Here's how the part is built. I have some questions about the finished solid (model axes, mm). Face numbers are marked on the shaded views. A direction names the side the tool comes from. Coordinates: 2 decimals unless noted, no trailing zeros. Order: outer loops, then holes, each group sorted by start corner. A loop starts at its lowest first (then second) coordinate and runs counter-clockwise, first axis right, second up. Notation, with made-up numbers: (6, 29.25) - (63, 29.25) arc R33 cw to (63, 64.25) - close; hole circle Ø3 at (-20, 34). An arc over 180 degrees is marked (long way). Answer as CSV lines item,"result". Start each with the question number.
Q1. For the marked faces 3 and 4, which set-ups out of +Z, -Z, +X, -X, +Y, -Y let a thin tool reach every point of the face, with its end or its side?
Q2. Suppose I cut it at B-B (z = -20). Please give me the cut outline in (x, y).
Q3. Thinking about a two-plate mould opening in Z: for the marked faces 1 and 2, which applies, released by +Z, released by -Z, zero draft, split by the parting line, or undercut?
Q4. Suppose I cut it at C-C (x = -1.5). Please give me the cut outline in (y, z).
Q5. I need wall thicknesses on line 1 (Z direction, x = 54, y = 0.75); line 2 (Z direction, x = 26, y = 3.75); line 3 (Z direction, x = -33, y = 3.5). Which ranges of each line are inside material? Lowest first, please.
Q6. Suppose I cut it at A-A (x = -64.5). Please give me the cut outline in (y, z), then the cut area to 3 significant figures.
Q7. Suppose I cut it at D-D (x = 125). Please give me the cut outline in (y, z) (3 decimals).
Q8. For pin 1 Ø6 at (x, z) = (143.5, -4.5) entering from -Y; pin 2 Ø1.9 at (y, z) = (3.5, 83.5) entering from +X; pin 3 Ø5 at (x, z) = (125.5, -4) entering from +Y, each with a flat end and sliding along its axis, tell me the tip position at first contact or that it passes through.
from build123d import *

# Parameters (mm, degrees)
SALIENTE_EXTRUIR1_DEPTH = 6.35
CROQUIS2_R              = 1.825
CROQUIS2_W              = 63.849825594
CROQUIS2_H              = 10
CROQUIS2_W_2            = 24.299825594
CORTAR_EXTRUIR1_DEPTH   = 220.409920137
CROQUIS4_W              = 45
CROQUIS4_H              = 84.1
CORTAR_EXTRUIR3_DEPTH   = 1.5
CROQUIS5_R              = 1.75
CORTAR_EXTRUIR4_DEPTH   = 220.371632292
CROQUIS7_W              = 45
CROQUIS7_H              = 2.275
CORTAR_EXTRUIR5_DEPTH   = 1.5
CROQUIS9_W              = 125
CROQUIS9_H              = 146
CORTAR_EXTRUIR7_DEPTH   = 4.3
CROQUIS10_R             = 2.8
CORTAR_EXTRUIR8_DEPTH   = 4.35
CORTAR_EXTRUIR12_DEPTH  = 220.409920137
CORTAR_EXTRUIR15_DEPTH  = 1.5
CROQUIS19_W             = 7.395174406
CROQUIS19_H             = 10
CORTAR_EXTRUIR16_DEPTH  = 220.409920137
CROQUIS20_W             = 60.600000004
CROQUIS20_H             = 97.5
CORTAR_EXTRUIR17_DEPTH  = 4
CROQUIS21_R             = 1.825
CORTAR_EXTRUIR18_DEPTH  = 220.354486059
CROQUIS25_W             = 35.4
CROQUIS25_H             = 12
CORTAR_EXTRUIR21_DEPTH  = 220.409920137
CORTAR_EXTRUIR22_DEPTH  = 220.36016173
CROQUIS28_R             = 1.825
CORTAR_EXTRUIR24_DEPTH  = 220.409920137


with BuildPart() as part:
    # Croquis1 → Saliente-Extruir1 (new body)
    with BuildSketch(Plane(origin=(0, 0, 0), x_dir=(1, 0, 0), z_dir=(0, 1, 0))):
        with BuildLine():
            Line((0, 0), (200, 0))
            Line((200, 0), (200, 15.2))
            ThreePointArc((200, 15.2), (197.701163079, 20.938172036), (191.9990235, 23.3249845))
            ThreePointArc((191.9990235, 23.3249845), (148.666739026, 44.032184001), (120.7781513, 83.1307986))
            ThreePointArc((120.7781513, 83.1307986), (113.982057966, 88.196272982), (105.7, 90))
            Line((105.7, 90), (0, 90))
            Line((0, 90), (-79, 90))
            ThreePointArc((-79, 90), (-84.638146896, 87.675499941), (-86.999825594, 82.052824894))
            Line((-86.999825594, 82.052824894), (-86.999825594, 41.494023494))
            ThreePointArc((-86.999825594, 41.494023494), (-92.052704294, 29.329564667), (-102.353503833, 21.119864881))
            ThreePointArc((-102.353503833, 21.119864881), (-108.040391417, 18.79326931), (-110.4, 13.12))
            Line((-110.4, 13.12), (-110.4, 0))
            Line((-110.4, 0), (0, 0))
        make_face()
    extrude(amount=SALIENTE_EXTRUIR1_DEPTH)

    # Simetría2: part across plane


with BuildPart() as part_1:
    add(part.part)
    add(part.part.mirror(Plane(origin=(0, 6.35, 0), x_dir=(1, 0, 0), z_dir=(0, 0, -1))))

    # Croquis2 → Cortar-Extruir1 (cut, through all)
    with BuildSketch(Plane(origin=(0, 6.35, 0), x_dir=(1, 0, 0), z_dir=(0, 1, 0))):
        with Locations(Location((68.5, 81.35, 0), (0, 0, 270))):
            Circle(CROQUIS2_R)
        with Locations(Location((-16.05, 81.35, 0), (0, 0, 270))):
            Circle(CROQUIS2_R)
        with Locations(Location((68.5, -81.35, 0), (0, 0, 90))):
            Circle(CROQUIS2_R)
        with Locations(Location((-16.05, -81.35, 0), (0, 0, 90))):
            Circle(CROQUIS2_R)
        with Locations((29.925087203, -81.35)):
            Rectangle(CROQUIS2_W, CROQUIS2_H)
        with Locations((-34.849912797, -81.35)):
            Rectangle(CROQUIS2_W_2, CROQUIS2_H)
        with Locations((87.299912797, -81.35)):
            Rectangle(CROQUIS2_W_2, CROQUIS2_H)
        with Locations((-34.849912797, 81.35)):
            Rectangle(CROQUIS2_W_2, CROQUIS2_H)
        with Locations((29.925087203, 81.35)):
            Rectangle(CROQUIS2_W, CROQUIS2_H)
        with Locations((87.299912797, 81.35)):
            Rectangle(CROQUIS2_W_2, CROQUIS2_H)
    extrude(amount=-CORTAR_EXTRUIR1_DEPTH, mode=Mode.SUBTRACT)

    # Croquis4 → Cortar-Extruir3 (cut)
    with BuildSketch(Plane(origin=(0, 6.35, 0), x_dir=(1, 0, 0), z_dir=(0, 1, 0))):
        with Locations((127.5, 0)):
            Rectangle(CROQUIS4_W, CROQUIS4_H)
    extrude(amount=-CORTAR_EXTRUIR3_DEPTH, mode=Mode.SUBTRACT)

    # Croquis5 → Cortar-Extruir4 (cut, through all)
    with BuildSketch(Plane(origin=(0, 4.85, 0), x_dir=(1, 0, 0), z_dir=(0, 1, 0))):
        with Locations(Location((147.25, 35.6, 0), (0, 0, 270))):
            Circle(CROQUIS5_R)
        with Locations(Location((107.75, 35.6, 0), (0, 0, 90))):
            Circle(CROQUIS5_R)
        with Locations(Location((147.25, -35.6, 0), (0, 0, 90))):
            Circle(CROQUIS5_R)
        with Locations(Location((107.75, -35.6, 0), (0, 0, 270))):
            Circle(CROQUIS5_R)
    extrude(amount=-CORTAR_EXTRUIR4_DEPTH, mode=Mode.SUBTRACT)

    # Croquis7 → Cortar-Extruir5 (cut)
    with BuildSketch(Plane(origin=(0, 6.35, 0), x_dir=(1, 0, 0), z_dir=(0, 1, 0))):
        with Locations((127.5, 43.1875)):
            Rectangle(CROQUIS7_W, CROQUIS7_H)
    extrude(amount=-CORTAR_EXTRUIR5_DEPTH, mode=Mode.SUBTRACT)

    # Croquis9 → Cortar-Extruir7 (cut)
    with BuildSketch(Plane(origin=(0, 6.35, 0), x_dir=(1, 0, 0), z_dir=(0, 1, 0))):
        with Locations((36.10017441, 0)):
            Rectangle(CROQUIS9_W, CROQUIS9_H)
    extrude(amount=-CORTAR_EXTRUIR7_DEPTH, mode=Mode.SUBTRACT)

    # Croquis10 → Cortar-Extruir8 (cut)
    with BuildSketch(Plane.XZ):
        with Locations(Location((-16.05, 81.35, 0), (0, 0, 270))):
            Circle(CROQUIS10_R)
        with Locations(Location((-16.05, -81.35, 0), (0, 0, 90))):
            Circle(CROQUIS10_R)
        with Locations(Location((68.5, -81.35, 0), (0, 0, 270))):
            Circle(CROQUIS10_R)
        with Locations(Location((68.5, 81.35, 0), (0, 0, 90))):
            Circle(CROQUIS10_R)
    extrude(amount=-CORTAR_EXTRUIR8_DEPTH, mode=Mode.SUBTRACT)

    # Croquis16 → Cortar-Extruir12 (cut, through all)
    with BuildSketch(Plane(origin=(0, 6.35, 0), x_dir=(1, 0, 0), z_dir=(0, 1, 0))):
        Polygon((-86.999825594, 41.494023494), (-110.4, 41.494023494), (-110.4, 13.12), (-110.4, -13.12), (-110.4, -41.494023494), (-86.999825594, -41.494023494), align=None)
    extrude(amount=-CORTAR_EXTRUIR12_DEPTH, mode=Mode.SUBTRACT)

    # Croquis18 → Cortar-Extruir15 (cut)
    with BuildSketch(Plane(origin=(0, 6.35, 0), x_dir=(1, 0, 0), z_dir=(0, 1, 0))):
        Polygon((105, 44.325), (103, 44.325), (103, -44.05), (150, -44.05), (150, -42.05), (105, -42.05), align=None)
    extrude(amount=-CORTAR_EXTRUIR15_DEPTH, mode=Mode.SUBTRACT)

    # Croquis19 → Cortar-Extruir16 (cut, through all)
    with BuildSketch(Plane(origin=(0, 6.35, 0), x_dir=(1, 0, 0), z_dir=(0, 1, 0))):
        with Locations((-5.697412797, 81.35)):
            Rectangle(CROQUIS19_W, CROQUIS19_H)
        with Locations((-5.697412797, -81.35)):
            Rectangle(CROQUIS19_W, CROQUIS19_H)
    extrude(amount=-CORTAR_EXTRUIR16_DEPTH, mode=Mode.SUBTRACT)

    # Croquis20 → Cortar-Extruir17 (cut)
    with BuildSketch(Plane(origin=(0, 6.35, 0), x_dir=(1, 0, 0), z_dir=(0, 1, 0))):
        with Locations((-56.699825592, 0)):
            Rectangle(CROQUIS20_W, CROQUIS20_H)
    extrude(amount=-CORTAR_EXTRUIR17_DEPTH, mode=Mode.SUBTRACT)

    # Croquis21 → Cortar-Extruir18 (cut, through all)
    with BuildSketch(Plane(origin=(0, 2.35, 0), x_dir=(1, 0, 0), z_dir=(0, 1, 0))):
        with Locations(Location((-77.999825594, 41.75, 0), (0, 0, 270))):
            Circle(CROQUIS21_R)
        with Locations(Location((-35.999825594, 41.75, 0), (0, 0, 270))):
            Circle(CROQUIS21_R)
        with Locations(Location((-35.999825594, -41.75, 0), (0, 0, 270))):
            Circle(CROQUIS21_R)
        with Locations(Location((-77.999825594, -41.75, 0), (0, 0, 270))):
            Circle(CROQUIS21_R)
    extrude(amount=-CORTAR_EXTRUIR18_DEPTH, mode=Mode.SUBTRACT)

    # Croquis25 → Cortar-Extruir21 (cut, through all)
    with BuildSketch(Plane.XZ):
        with Locations((-49.699825594, 58.76)):
            Rectangle(CROQUIS25_W, CROQUIS25_H)
        with Locations((-49.699825594, -58.76)):
            Rectangle(CROQUIS25_W, CROQUIS25_H)
    extrude(amount=-CORTAR_EXTRUIR21_DEPTH, mode=Mode.SUBTRACT)

    # Croquis26 → Cortar-Extruir22 (cut, through all)
    with BuildSketch(Plane(origin=(0, 2.05, 0), x_dir=(1, 0, 0), z_dir=(0, 1, 0))):
        Polygon((-11.39982559, 71.5), (-11.39982559, 58), (-24.89982559, 58), (-24.89982559, -58), (-11.39982559, -58), (-11.39982559, -71.5), (83.60017441, -71.5), (83.60017441, -58), (97.10017441, -58), (97.10017441, 58), (83.60017441, 58), (83.60017441, 71.5), align=None)
    extrude(amount=-CORTAR_EXTRUIR22_DEPTH, mode=Mode.SUBTRACT)

    # Croquis28 → Cortar-Extruir24 (cut, through all)
    with BuildSketch(Plane(origin=(0, 6.35, 0), x_dir=(1, 0, 0), z_dir=(0, 1, 0))):
        with Locations(Location((-75.199825594, -62.81, 0), (0, 0, 270))):
            Circle(CROQUIS28_R)
        with Locations(Location((-58.699825594, -86, 0), (0, 0, 270))):
            Circle(CROQUIS28_R)
        with Locations(Location((-75.199825594, 62.81, 0), (0, 0, 90))):
            Circle(CROQUIS28_R)
        with Locations(Location((-58.699825594, 86, 0), (0, 0, 90))):
            Circle(CROQUIS28_R)
    extrude(amount=-CORTAR_EXTRUIR24_DEPTH, mode=Mode.SUBTRACT)


solid = part_1.part
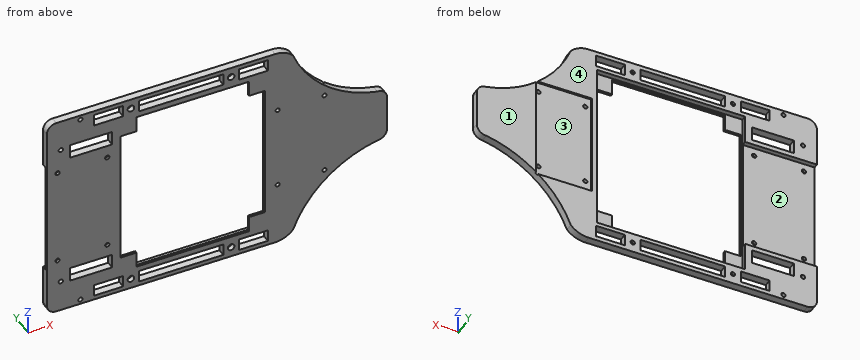
Here are the results:
1,face 3,"+Y"
1,face 4,"+Z, -Z, +X, -X, +Y"
2,outline,"(-87, 0) - (-24.9, 0) - (-24.9, 2.05) - (-26.4, 2.05) - (-26.4, 2.35) - (-87, 2.35) - close; (97.1, 0) - (198.49, 0) - (198.49, 6.35) - (150, 6.35) - (150, 4.85) - (103, 4.85) - (103, 6.35) - (98.6, 6.35) - (98.6, 2.05) - (97.1, 2.05) - close"
3,face 1,"zero draft"
3,face 2,"undercut"
4,outline,"(0, -90) - (6.35, -90) - (6.35, -86.35) - (0, -86.35) - close; (0, -76.35) - (6.35, -76.35) - (6.35, -73) - (2.05, -73) - (2.05, -71.5) - (0, -71.5) - close; (0, 71.5) - (2.05, 71.5) - (2.05, 73) - (6.35, 73) - (6.35, 76.35) - (0, 76.35) - close; (0, 86.35) - (6.35, 86.35) - (6.35, 90) - (0, 90) - close"
5,line 1,"z = -90 to -86.35, -76.35 to -71.5, 71.5 to 76.35, 86.35 to 90"
5,line 2,"z = -90 to -86.35, -76.35 to -73, 73 to 76.35, 86.35 to 90"
5,line 3,"z = -90 to -86.35, -76.35 to -64.76, -52.76 to -48.75, 48.75 to 52.76, 64.76 to 76.35, 86.35 to 90"
6,outline,"(0, -90) - (6.35, -90) - (6.35, -64.76) - (0, -64.76) - close; (0, -52.76) - (6.35, -52.76) - (6.35, -48.75) - (2.35, -48.75) - (2.35, 48.75) - (6.35, 48.75) - (6.35, 52.76) - (0, 52.76) - close; (0, 64.76) - (6.35, 64.76) - (6.35, 90) - (0, 90) - close"
6,area,"601 mm²"
7,outline,"(0, -73.695) - (6.35, -73.695) - (6.35, -44.325) - (4.85, -44.325) - (4.85, 44.05) - (6.35, 44.05) - (6.35, 73.695) - (0, 73.695) - close"
8,pin 1,"stops at y = 0"
8,pin 2,"stops at x = 121"
8,pin 3,"stops at y = 4.85"
